Geometry: final body of the model. Coordinates: model frame, mm. Face numbers are marked on the shaded views. Coordinates: 2 decimals unless noted, no trailing zeros. Write each loop counter-clockwise with the first axis right and the second up, starting at its lowest first coordinate (ties: lowest second). Pieces come first, ordered by that corner, then holes. Notation, with made-up numbers: M -2,-22 L 41,-22 A38 ccw 41,17 Z; hole C 55.25,-18.75 d11. An arc over 180 degrees is marked long. Write item = value, one per line. Start each with the question number.
Item 1: Section D-D on x = -36. Output: boundary loops of the cut face in (y, z), plus the area to 3 significant figures.
Item 2: Section C-C on x = 6.5. Output: boundary loops of the cut face in (y, z).
Item 3: Section A-A on z = 0. Output: boundary loops of the cut face in (x, y).
Item 4: Pull-direction query (Z, two-part tool) for the marked faces 1 and 2; classes: +Z half, -Z half, draft (parallel to the pull), parting line (faces both ways), or undercut.
Item 5: Ray query, L1, parallel to X at y = 5.5, z = 2.5; L2, parallel to X at y = -4, z = -1.5; L3, parallel to Y at x = -14, z = -0.25. Return the intervals inside material, ascending. Write a range as [from, to].
Item 6: First-contact query: pin 1 Ø3 at (x, z) = (13.5, 3) entering from +Y; pin 2 Ø2 at (x, z) = (-3.5, -1) entering from -Y. Flat tips, straight axial feed; report the tip coordinate or a pass-through.
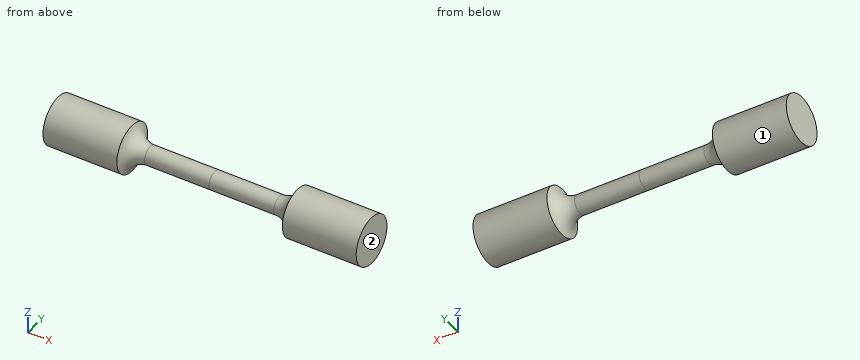
from build123d import *


with BuildPart() as part:
    # Sketch → Revolution (revolve)
    with BuildSketch(Plane.XY):
        with BuildLine():
            Line((-42.398979, 6.5), (-42.398979, 0))
            Line((0, 0), (-42.398979, 0))
            Line((0, 2.5), (0, 0))
            Line((-17.5, 2.5), (0, 2.5))
            ThreePointArc((-22.398979, 6.5), (-20.662278, 3.627017), (-17.5, 2.5))
            Line((-42.398979, 6.5), (-22.398979, 6.5))
        make_face()
    revolution = revolve(axis=Axis((0, 0, 0), (1, 0, 0)))

    # Mirrored: Revolution across Sketch V_Axis
    add(revolution.mirror(Plane(origin=(0, 0, 0), x_dir=(0, 0, 1), z_dir=(1, 0, 0))))


solid = part.part
Responses:
q1.outline = C 0,0 d13
q1.area = 133 mm²
q2.outline = C 0,0 d5
q3.outline = M -42.4,-6.5 L -22.4,-6.5 A5 cw -17.5,-2.5 L 17.5,-2.5 A5 cw 22.4,-6.5 L 42.4,-6.5 L 42.4,6.5 L 22.4,6.5 A5 cw 17.5,2.5 L -17.5,2.5 A5 cw -22.4,6.5 L -42.4,6.5 Z
q4.face_1 = parting line
q4.face_2 = draft
q5.L1 = [-42.4, -22.28], [22.28, 42.4]
q5.L2 = [-42.4, -21.32], [21.32, 42.4]
q5.L3 = [-2.49, 2.49]
q6.pin_1 = 2
q6.pin_2 = -2.5
